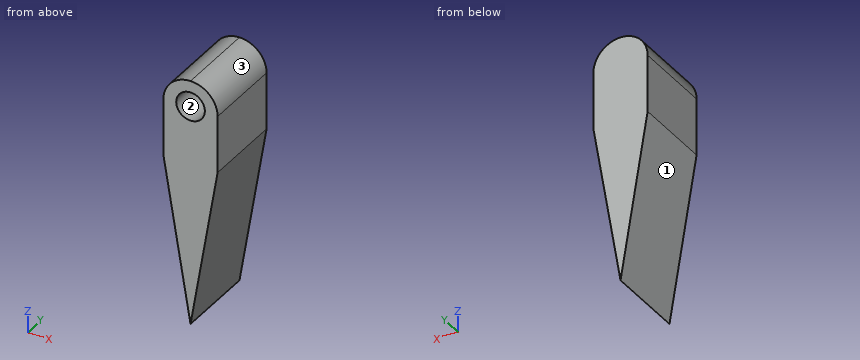
from build123d import *

# Parameters (mm, degrees)
BOSS_EXTRUDE1_DEPTH = 19.05
FILLET1_R           = 6.35
SKETCH3_R           = 3.353621891
CUT_EXTRUDE1_DEPTH  = 12.7


with BuildPart() as part:
    # Sketch1 → Boss-Extrude1 (new body)
    with BuildSketch(Plane(origin=(0, 0, 0), x_dir=(1, 0, 0), z_dir=(0, 1, 0))):
        Polygon((0, 38.1), (-6.35, 0), (-6.35, -19.685), (6.35, -19.685), (6.35, 0), align=None)
    extrude(amount=BOSS_EXTRUDE1_DEPTH)

    # Fillet1
    fillet1_edges = [part.edges().sort_by_distance(p)[0] for p in [
        (-6.35, 9.525, 19.685),
        (6.35, 9.525, 19.685),
    ]]
    fillet(fillet1_edges, radius=FILLET1_R - 0.0001)  # a hair under: the kernel refuses the full size

    # Sketch3 → Cut-Extrude1 (cut)
    with BuildSketch(Plane.XZ):
        with Locations(Location((0, 13.621650325, 0), (0, 0, 270))):
            Circle(SKETCH3_R)
    extrude(amount=-CUT_EXTRUDE1_DEPTH, mode=Mode.SUBTRACT)


solid = part.part
The listing builds one solid part. Answer for the finished solid, in the listing's coordinates (mm). Face numbers are marked on the shaded views. Give positions to 0.01 mm unless a question says otherwise; leave off trailing zeros. Write each loop counter-clockwise with the first axis right and the second up, starting at its lowest first coordinate (ties: lowest second). Pieces come first, ordered by that corner, then holes. Notation, with made-up numbers: (-27, 83) -> (16, 83) arc R22 cw to (16, 100) -> close; hole circle Ø4 at (66, 18.5). An arc over 180 degrees is marked (long way). One line per question, with ' | ' between items. Start each with the question number.
1. For a pull along X with two mould halves and no side action, classify the marked faces 1, 2 and 3 as pulls with the +X half, pulls with the -X half, needs draft (parallel to the pull), parting line crosses it, or undercut.
2. Section B-B (x = -2) is taken. Determine the outline of the cut face in (y, z).
3. Section D-D (z = -6) is taken. Determine the outline of the cut face in (x, y), plus the area to 3 significant figures.
4. Given pin 1 Ø1 at (x, y) = (4, 12.5) entering from +Z; pin 2 Ø4 at (y, z) = (10.5, -28) entering from -X; pin 3 Ø3.5 at (x, z) = (0, 14) entering from -Y; pin 4 Ø5 at (x, z) = (4.5, -27.5) entering from -Y, each flat-ended and moving along its own axis, determine where each tip first touches the part or whether it passes through.
5. Find the intervals of material crossed by probe 1 along X at (y, z) = (2, 14.5); probe 2 along X at (y, z) = (7.75, -33); probe 3 along X at (y, z) = (16, -13), in increasing order.
Response values:
1) face 1: pulls with the -X half | face 2: undercut | face 3: pulls with the +X half
2) outline: (0, -26.1) -> (19.05, -26.1) -> (19.05, 19.36) -> (0, 19.36) -> (0, 16.31) -> (12.7, 16.31) -> (12.7, 10.93) -> (0, 10.93) -> close
3) outline: (-5.35, 0) -> (5.35, 0) -> (5.35, 19.05) -> (-5.35, 19.05) -> close | area: 204 mm2
4) pin 1: z = 18.63 | pin 2: x = -2.02 | pin 3: y = 12.7 | pin 4: through
5) probe 1: -6.24 to -3.24, 3.24 to 6.24 | probe 2: -0.85 to 0.85 | probe 3: -4.18 to 4.18
